Here's how the part is built. I have some questions about the finished solid (model axes, mm). A direction names the side the tool comes from. Round coordinates to 2 decimals unless told otherwise and drop trailing zeros. Write each loop counter-clockwise with the first axis right and the second up, starting at its lowest first coordinate (ties: lowest second). Pieces come first, ordered by that corner, then holes. Notation, with made-up numbers: (29, 21) - (43, 21) arc R23 ccw to (43, 39) - close; hole circle Ø2 at (-38.5, 40.5). An arc over 180 degrees is marked (long way). Write item = value, one per line. Start each with the question number.
Item 1: If we section it at A-A (y = -360.5): Please give me the cut outline in (x, z), and give its area (3 significant figures).
Item 2: Thinking about a two-plate mould opening in Y: for faces 4 (the face through (14, -600, 0)), 5 (the face through (13.99, -68.49, -0.37)), 6 (the face through (13.99, -198.49, -0.37)), 7 (the face through (15, -296, 0)), which applies, pulls with the +Y half, pulls with the -Y half, needs draft (parallel to the pull), parting line crosses it, or undercut?
Item 3: Which directions (+Z, -Z, +X, -X, +Y, -Y) give clear straight access to the entire face, cutting with the end or side of a thin tool? Please do faces 1 (the face through (0, -296, 15)), 2 (the face through (-13, -296, 0)), 3 (the face through (13.99, -328.49, -0.37)).
Item 4: If I drill on line 1 along Y through (x, z) = (13.7, 0); line 2 along Z through (x, y) = (14.6, -320); line 3 along X through (y, z) = (-178.5, -3.75), over which ranges is the centre line in solid material (lowest first)? Write a range as [from, to].
Item 5: For P1, Ø15.5, axis at y = -190, z = 0, coming from the +X side, with a flat end and sliding along its axis, tell me the tip position at first contact or that it passes through.
Item 6: If we section it at B-B (x = 3): Please give me the cut outline in (y, z).
Item 7: If we section it at C-C (z = 0): Please give me the cut outline in (x, y).
Autodesk Inventor part; units mm, degrees
ref_plane "YZ Plane" through (0, 0, 0) normal (1, 0, 0) x (0, 1, 0)
ref_plane "XZ Plane" through (0, 0, 0) normal (0, 1, 0) x (-1, 0, 0)
ref_plane "XY Plane" through (0, 0, 0) normal (0, 0, 1) x (1, 0, 0)
sketch "Sketch9" plane through (0, 0, 0) normal (0, 1, 0) x (-1, 0, 0)
  line L0 (15, 15) -> (-15, 15)
  line L1 (-15, 15) -> (-15, -15)
  line L2 (-15, -15) -> (15, -15)
  line L3 (15, -15) -> (15, 15)
  line L4 (15, 15) -> (-15, -15) construction
  line L5 (-15, 15) -> (15, -15) construction
  line L6 (-13, 13) -> (13, 13)
  line L7 (13, 13) -> (13, -13)
  line L8 (13, -13) -> (-13, -13)
  line L9 (-13, -13) -> (-13, 13)
  point P0 (0, 0)
  dimension "d172" = 30
  dimension "d173" = 30
  dimension "d174" = 2
extrude "Extrusion3" add sketch "Sketch9" against normal blind 600
sketch "Sketch10" plane through (0, 0, 0) normal (1, 0, 0) x (0, 1, 0)
  line L0 (0, 15) -> (0, -15) construction
  line L1 (0, 15) -> (-600, 15) construction
  line L2 (-600, -15) -> (-600, 15) construction
  line L3 (0, -15) -> (-600, -15) construction
  line L4 (-68.5, 8.5) -> (-51.5, 8.5)
  line L5 (-51.5, 8.5) -> (-51.5, -8.5)
  line L6 (-51.5, -8.5) -> (-68.5, -8.5)
  line L7 (-68.5, -8.5) -> (-68.5, 8.5)
  line L8 (-68.5, 8.5) -> (-51.5, -8.5) construction
  line L9 (-51.5, 8.5) -> (-68.5, -8.5) construction
  line L10 (-198.5, 8.5) -> (-181.5, 8.5)
  line L11 (-181.5, 8.5) -> (-181.5, -8.5)
  line L12 (-181.5, -8.5) -> (-198.5, -8.5)
  line L13 (-198.5, -8.5) -> (-198.5, 8.5)
  line L14 (-198.5, 8.5) -> (-181.5, -8.5) construction
  line L15 (-181.5, 8.5) -> (-198.5, -8.5) construction
  line L16 (-328.5, 8.5) -> (-311.5, 8.5)
  line L17 (-311.5, 8.5) -> (-311.5, -8.5)
  line L18 (-311.5, -8.5) -> (-328.5, -8.5)
  line L19 (-328.5, -8.5) -> (-328.5, 8.5)
  line L20 (-328.5, 8.5) -> (-311.5, -8.5) construction
  line L21 (-311.5, 8.5) -> (-328.5, -8.5) construction
  circle A0 centre (-570, 0) radius 8.5
  line L22 (0, 0) -> (30, 0)
  circle A1 centre (-60, 0) radius 8.5
  circle A2 centre (-190, 0) radius 8.5
  circle A3 centre (-320, 0) radius 8.5
  dimension "d177" = 17
  dimension "d178" = 17
  dimension "d181" = 30
  dimension "d182" = 90
  dimension "d183" = 220
  dimension "d184" = 350
  dimension "d185" = 600
  dimension "d186" = 17
extrude "Extrusion4" cut sketch "Sketch10" along normal through all contours A1 | A2 | A3 | A0
properties part number "APN 754 FDS 1200 way tube 1" material "Stainless Steel"
Reply:
q1.outline = (-15, -15) - (15, -15) - (15, 15) - (-15, 15) - close; hole (-13, -13) - (13, -13) - (13, 13) - (-13, 13) - close
q1.area = 224 mm2
q2.face_4 = pulls with the -Y half
q2.face_5 = undercut
q2.face_6 = undercut
q2.face_7 = needs draft
q3.face_1 = +Z, +X, -X, +Y, -Y
q3.face_2 = +Y, -Y
q3.face_3 = +X
q4.line_1 = [-600, -578.5], [-561.5, -328.5], [-311.5, -198.5], [-181.5, -68.5], [-51.5, 0]
q4.line_2 = [-15, -8.5], [8.5, 15]
q4.line_3 = [-15, -13], [13, 15]
q5.P1 = -13
q6.outline = (-600, -15) - (0, -15) - (0, -13) - (-600, -13) - close; (-600, 13) - (0, 13) - (0, 15) - (-600, 15) - close
q7.outline = (-15, -600) - (-13, -600) - (-13, 0) - (-15, 0) - close; (13, -600) - (15, -600) - (15, -578.5) - (13, -578.5) - close; (13, -561.5) - (15, -561.5) - (15, -328.5) - (13, -328.5) - close; (13, -311.5) - (15, -311.5) - (15, -198.5) - (13, -198.5) - close; (13, -181.5) - (15, -181.5) - (15, -68.5) - (13, -68.5) - close; (13, -51.5) - (15, -51.5) - (15, 0) - (13, 0) - close
